The listing builds one solid part. Answer for the finished solid, in the listing's coordinates (mm). Face numbers are marked on the shaded views. A direction names the side the tool comes from. Coordinates: 2 decimals unless noted, no trailing zeros. Order: outer loops, then holes, each group sorted by start corner. A loop starts at its lowest first (then second) coordinate and runs counter-clockwise, first axis right, second up. Notation, with made-up numbers: (14.25, 11.25) -> (70.25, 11.25) arc R22 ccw to (70.25, 45.25) -> close; hole circle Ø1 at (15.25, -27.75). An arc over 180 degrees is marked (long way). Write item = value, one per line.
from build123d import *

# Parameters (mm, degrees)
OREJA_ANTERIOR_DEPTH         = 3
OREJA_POSTERIOR_DEPTH        = 3
SKETCH3_W                    = 18
SKETCH3_H                    = 8
PUENTE_DEPTH                 = 25
SKETCH5_R                    = 2.6
AGUJERO_EJE_DESVIACION_DEPTH = 1000


with BuildPart() as part:
    # Sketch1 → Oreja_anterior (new body)
    with BuildSketch(Plane.XY.offset(-12.5)):
        with BuildLine():
            Line((7, 0), (7, -16))
            ThreePointArc((7, -16), (0, -23), (-7, -16))
            Line((-7, -16), (-7, 0))
            ThreePointArc((-7, 0), (0, 7), (7, 0))
        make_face()
    extrude(amount=OREJA_ANTERIOR_DEPTH)



with BuildPart() as body_2:
    # Sketch2 → Oreja_posterior (new body)
    with BuildSketch(Plane.XY.offset(9.5)):
        with BuildLine():
            Line((7, 0), (7, -16))
            ThreePointArc((7, -16), (0, -23), (-7, -16))
            Line((-7, -16), (-7, 0))
            ThreePointArc((-7, 0), (0, 7), (7, 0))
        make_face()
    extrude(amount=OREJA_POSTERIOR_DEPTH)


with BuildPart() as part_1:
    add(part.part)

    add(body_2.part)  # Puente merges body 2
    # Sketch3 → Puente (add)
    with BuildSketch(Plane.XY.offset(-12.5)):
        with Locations((0, -19)):
            Rectangle(SKETCH3_W, SKETCH3_H)
    extrude(amount=PUENTE_DEPTH)

    # Sketch4 → Brida_mano (revolve)
    with BuildSketch(Plane.XY, mode=Mode.PRIVATE) as brida_mano_sk:
        Polygon((0, -21), (11, -21), (24, -22), (24, -27), (11, -27), (0, -27), align=None)
    revolve(brida_mano_sk.sketch.rotate(Axis((0, -31, 0), (0, 1, 0)), 90), axis=Axis((0, -31, 0), (0, 1, 0)))

    # Sketch5 → Agujero_eje_desviacion (cut, symmetric)
    with BuildSketch(Plane.XY):
        Circle(SKETCH5_R)
    extrude(amount=AGUJERO_EJE_DESVIACION_DEPTH, both=True, mode=Mode.SUBTRACT)


solid = part_1.part
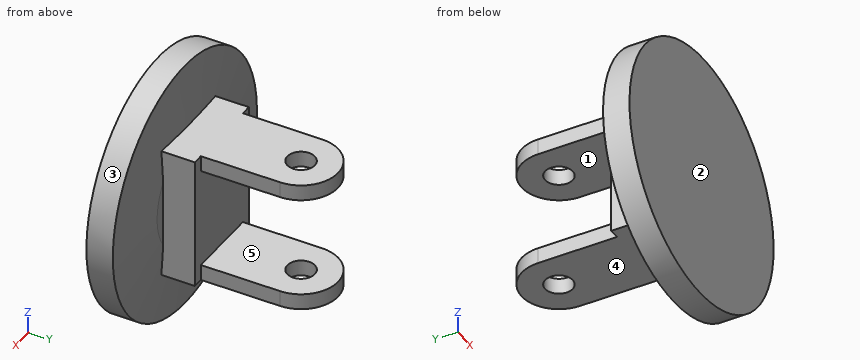
Q1. Section D-D, the plane y = -19 is taken. Give the vertices of the cut face in (x, z).
The answers:
outline = (-9, -12.5) -> (9, -12.5) -> (9, 12.5) -> (-9, 12.5) -> close
Q2. Section B-B, the plane x = 0 is taken. Give the vertices of the cut face in (y, z).
The answers:
outline = (-27, -24) -> (-22, -24) -> (-21.12, -12.5) -> (-2.6, -12.5) -> (-2.6, -9.5) -> (-15, -9.5) -> (-15, 9.5) -> (-2.6, 9.5) -> (-2.6, 12.5) -> (-21.12, 12.5) -> (-22, 24) -> (-27, 24) -> close; (2.6, -12.5) -> (7, -12.5) -> (7, -9.5) -> (2.6, -9.5) -> close; (2.6, 9.5) -> (7, 9.5) -> (7, 12.5) -> (2.6, 12.5) -> close
Q3. A tool of negligible diameter and unlimited length cuts with its end or side. For the marked faces 1 and 2, from which of +Z, -Z, +X, -X, +Y, -Y can it reach the whole face along a straight path? Write none if from no direction.
The answers:
face_1 = +X, -X, +Y
face_2 = +Z, -Z, +X, -X, -Y
Q4. The mould has two halves that part along Z. Classify the marked faces 3, 4 and 5: released by +Z, released by -Z, zero draft, split by the parting line, or undercut.
The answers:
face_3 = split by the parting line
face_4 = released by -Z
face_5 = undercut
Q5. Section A-A, the plane y = -10.5 is taken. Give the vertices of the cut face in (x, z), plus the area to 3 significant figures.
The answers:
outline = (-7, -12.5) -> (7, -12.5) -> (7, -9.5) -> (-7, -9.5) -> close; (-7, 9.5) -> (7, 9.5) -> (7, 12.5) -> (-7, 12.5) -> close
area = 84.0 mm2
Q6. Find the intervals of material crossed by line 1 along Z through (x, y) = (-5.5, -4); line 2 along Y through (x, z) = (0, 10.2); line 3 along X through (y, z) = (-17.5, -9), in increasing order.
The answers:
line_1 = -12.5 to -9.5, 9.5 to 12.5
line_2 = -27 to -2.6, 2.6 to 7
line_3 = -9 to 9
Q7. Section C-C, the plane z = 0 is taken. Give the vertices of the cut face in (x, y).
The answers:
outline = (-24, -27) -> (24, -27) -> (24, -22) -> (11, -21) -> (9, -21) -> (9, -15) -> (-9, -15) -> (-9, -21) -> (-11, -21) -> (-24, -22) -> close
Q8. Each of these flat-tipped pins is pushed along its axis until it touches: pin 1 Ø1.9 at (y, z) = (-18.5, 6) entering from -X; pin 2 Ø12 at (y, z) = (-22, -14) entering from -X; pin 3 Ø4.5 at (x, y) = (0, 0) entering from -Z; pin 4 Ø5.5 at (x, y) = (0.5, -10.5) entering from +Z. Where does it stop, or does it pass through?
The answers:
pin_1 = -9
pin_2 = -22.63
pin_3 = through
pin_4 = 12.5
